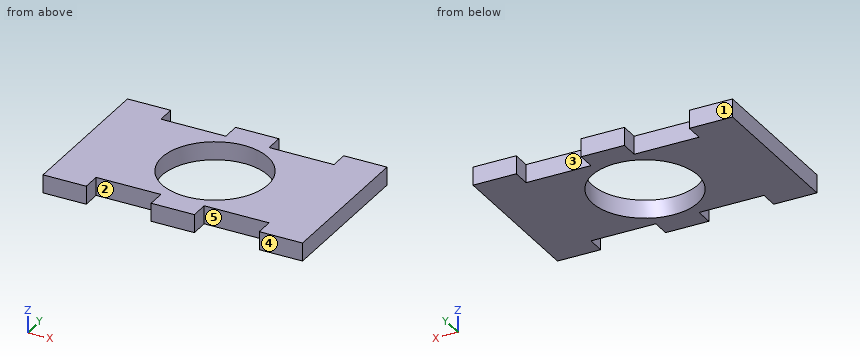
from build123d import *

# Parameters (mm, degrees)
SKETCH1_W           = 76.2
SKETCH1_H           = 35.2
BOSS_EXTRUDE1_DEPTH = 5.334
SKETCH2_R           = 15.55
CUT_EXTRUDE1_DEPTH  = 43.306282701
SKETCH3_W           = 12.7
SKETCH3_H           = 5.334
BOSS_EXTRUDE2_DEPTH = 5.334
SKETCH4_W           = 12.7
SKETCH4_H           = 5.334
BOSS_EXTRUDE3_DEPTH = 5.334


with BuildPart() as part:
    # Sketch1 → Boss-Extrude1 (new body)
    with BuildSketch(Plane.XY):
        Rectangle(SKETCH1_W, SKETCH1_H)
    extrude(amount=-BOSS_EXTRUDE1_DEPTH)

    # Sketch2 → Cut-Extrude1 (cut, through all)
    with BuildSketch(Plane.XY):
        Circle(SKETCH2_R)
    extrude(amount=-CUT_EXTRUDE1_DEPTH, mode=Mode.SUBTRACT)

    # Sketch3 → Boss-Extrude2 (add)
    with BuildSketch(Plane(origin=(0, 17.6, 0), x_dir=(1, 0, 0), z_dir=(0, 1, 0))):
        with Locations((-31.75, 2.667)):
            Rectangle(SKETCH3_W, SKETCH3_H)
        with Locations((0, 2.667)):
            Rectangle(SKETCH3_W, SKETCH3_H)
        with Locations((31.75, 2.667)):
            Rectangle(SKETCH3_W, SKETCH3_H)
    extrude(amount=BOSS_EXTRUDE2_DEPTH)

    # Sketch4 → Boss-Extrude3 (add)
    with BuildSketch(Plane.XZ.offset(17.6)):
        with Locations((-31.75, -2.667)):
            Rectangle(SKETCH4_W, SKETCH4_H)
        with Locations((0, -2.667)):
            Rectangle(SKETCH4_W, SKETCH4_H)
        with Locations((31.75, -2.667)):
            Rectangle(SKETCH4_W, SKETCH4_H)
    extrude(amount=BOSS_EXTRUDE3_DEPTH)


solid = part.part
The model under review builds one solid part; all positions refer to its coordinate system, in mm. Face numbers are marked on the shaded views. A direction names the side the tool comes from. Round coordinates to 2 decimals unless told otherwise and drop trailing zeros. Order: outer loops, then holes, each group sorted by start corner. A loop starts at its lowest first (then second) coordinate and runs counter-clockwise, first axis right, second up. Notation, with made-up numbers: (81.25, 10.25) -> (122.25, 10.25) arc R14 ccw to (122.25, 27.25) -> close; hole circle Ø2 at (72.25, 28.25). An arc over 180 degrees is marked (long way). Use CSV: the item, a comma, the result in double quotes. Start each with the question number.
(1) Consider section C-C on z = -3.2. Write out the cut boundary in (x, y), and give its area (3 significant figures).
(2) Insertion check: pin 1 (4 mm diameter, centred on x = -21, y = -11.5, fed in from +Z); pin 2 (1.6 mm diameter, centred on x = -11.5, z = -2.5, fed in from +Y). Each pin has a flat end and moves straight along its axis. Give the tip position at first contact, or say it passes through.
(3) Mouldability with a two-part tool opening along X and no side actions: class the marked faces 1 and 2 as pulls with the +X half, pulls with the -X half, needs draft (parallel to the pull), parting line crosses it, or undercut.
(4) Consider section D-D on x = -22. Write out the cut boundary in (y, z), and give its area (3 significant figures).
(5) Consider section B-B on x = 0. Write out the cut boundary in (y, z).
(6) Wall thickness on probe 1 along X at (y, z) = (18, -0.35); probe 2 along Y at (x, z) = (-0.5, -2.9); probe 3 along Y at (x, z) = (-21, -4.4): over which ranges is each line inside the solid? List them lowest first. Write a range as from..to.
(7) Consider section A-A on y = 0. Write out the cut boundary in (x, z).
(8) Tool access review of the marked faces 3, 4 and 5: name each direction out of +Z, -Z, +X, -X, +Y, -Y from which nothing blocks a thin tool from reaching the whole face with its end or side.
Responses:
1,outline,"(-38.1, -22.93) -> (-25.4, -22.93) -> (-25.4, -17.6) -> (-6.35, -17.6) -> (-6.35, -22.93) -> (6.35, -22.93) -> (6.35, -17.6) -> (25.4, -17.6) -> (25.4, -22.93) -> (38.1, -22.93) -> (38.1, 22.93) -> (25.4, 22.93) -> (25.4, 17.6) -> (6.35, 17.6) -> (6.35, 22.93) -> (-6.35, 22.93) -> (-6.35, 17.6) -> (-25.4, 17.6) -> (-25.4, 22.93) -> (-38.1, 22.93) -> close; hole circle Ø31.1 at (0, 0)"
1,area,"2,330 mm²"
2,pin 1,"z = 0"
2,pin 2,"y = 17.6"
3,face 1,"needs draft"
3,face 2,"undercut"
4,outline,"(-17.6, -5.33) -> (17.6, -5.33) -> (17.6, 0) -> (-17.6, 0) -> close"
4,area,"188 mm²"
5,outline,"(-22.93, -5.33) -> (-15.55, -5.33) -> (-15.55, 0) -> (-22.93, 0) -> close; (15.55, -5.33) -> (22.93, -5.33) -> (22.93, 0) -> (15.55, 0) -> close"
6,probe 1,"-38.1..-25.4, -6.35..6.35, 25.4..38.1"
6,probe 2,"-22.93..-15.54, 15.54..22.93"
6,probe 3,"-17.6..17.6"
7,outline,"(-38.1, -5.33) -> (-15.55, -5.33) -> (-15.55, 0) -> (-38.1, 0) -> close; (15.55, -5.33) -> (38.1, -5.33) -> (38.1, 0) -> (15.55, 0) -> close"
8,face 3,"+Z, -Z, +Y"
8,face 4,"+Z, -Z, +X, -X, -Y"
8,face 5,"+Z, -Z, -Y"
